from build123d import *

# Parameters (mm, degrees)
SKETCH1_W           = 4
SKETCH1_H           = 21
BOSS_EXTRUDE1_DEPTH = 4
CUT_EXTRUDE1_REACH  = 174.587
SKETCH3_W           = 34
SKETCH3_H           = 4
SKETCH3_W_2         = 46
SKETCH3_W_3         = 24


with BuildPart() as part:
    # Sketch1 → Boss-Extrude1 (new body)
    with BuildSketch(Plane(origin=(0, 0, 0), x_dir=(1, 0, 0), z_dir=(0, 1, 0))):
        with BuildLine():
            Line((-170, -29.5), (170, -29.5))
            Line((170, -29.5), (170, 29.5))
            Line((170, 29.5), (112, 29.5))
            Line((112, 29.5), (112, 25.5))
            Line((112, 25.5), (78, 25.5))
            Line((78, 25.5), (78, 29.5))
            Line((78, 29.5), (52.1, 29.5))
            Line((52.1, 29.5), (52.1, 27.5))
            ThreePointArc((52.1, 27.5), (50.5, 25.9), (48.9, 27.5))
            Line((48.9, 27.5), (48.9, 29.5))
            Line((48.9, 29.5), (23, 29.5))
            Line((23, 29.5), (23, 25.5))
            Line((23, 25.5), (-23, 25.5))
            Line((-23, 25.5), (-23, 29.5))
            Line((-23, 29.5), (-48.9, 29.5))
            Line((-48.9, 29.5), (-48.9, 27.5))
            ThreePointArc((-48.9, 27.5), (-50.5, 25.9), (-52.1, 27.5))
            Line((-52.1, 27.5), (-52.1, 29.5))
            Line((-52.1, 29.5), (-78, 29.5))
            Line((-78, 29.5), (-78, 25.5))
            Line((-78, 25.5), (-112, 25.5))
            Line((-112, 25.5), (-112, 29.5))
            Line((-112, 29.5), (-170, 29.5))
            Line((-170, 29.5), (-170, -29.5))
        make_face()
        with Locations((-148, -2)):
            Rectangle(SKETCH1_W, SKETCH1_H, mode=Mode.SUBTRACT)
        with Locations((148, -2)):
            Rectangle(SKETCH1_W, SKETCH1_H, mode=Mode.SUBTRACT)
    extrude(amount=BOSS_EXTRUDE1_DEPTH)

    # Sketch3 → Cut-Extrude1 (cut, up to next)
    with BuildSketch(Plane.XZ, mode=Mode.PRIVATE) as cut_extrude1_sk1:
        with Locations((-95, 27.5)):
            Rectangle(SKETCH3_W, SKETCH3_H)
    cut_extrude1_tool1 = extrude(cut_extrude1_sk1.sketch, amount=-CUT_EXTRUDE1_REACH, mode=Mode.PRIVATE) & part.part
    # Sketch3 → Cut-Extrude1 (cut, up to next)
    with BuildSketch(Plane.XZ, mode=Mode.PRIVATE) as cut_extrude1_sk2:
        with Locations((0, 27.5)):
            Rectangle(SKETCH3_W_2, SKETCH3_H)
    cut_extrude1_tool2 = extrude(cut_extrude1_sk2.sketch, amount=-CUT_EXTRUDE1_REACH, mode=Mode.PRIVATE) & part.part
    # Sketch3 → Cut-Extrude1 (cut, up to next)
    with BuildSketch(Plane.XZ, mode=Mode.PRIVATE) as cut_extrude1_sk3:
        with Locations((95, 27.5)):
            Rectangle(SKETCH3_W, SKETCH3_H)
    cut_extrude1_tool3 = extrude(cut_extrude1_sk3.sketch, amount=-CUT_EXTRUDE1_REACH, mode=Mode.PRIVATE) & part.part
    # Sketch3 → Cut-Extrude1 (cut, up to next)
    with BuildSketch(Plane.XZ, mode=Mode.PRIVATE) as cut_extrude1_sk4:
        with Locations((-158, -27.5)):
            Rectangle(SKETCH3_W_3, SKETCH3_H)
    cut_extrude1_tool4 = extrude(cut_extrude1_sk4.sketch, amount=-CUT_EXTRUDE1_REACH, mode=Mode.PRIVATE) & part.part
    # Sketch3 → Cut-Extrude1 (cut, up to next)
    with BuildSketch(Plane.XZ, mode=Mode.PRIVATE) as cut_extrude1_sk5:
        with Locations((158, -27.5)):
            Rectangle(SKETCH3_W_3, SKETCH3_H)
    cut_extrude1_tool5 = extrude(cut_extrude1_sk5.sketch, amount=-CUT_EXTRUDE1_REACH, mode=Mode.PRIVATE) & part.part
    add(cut_extrude1_tool1.solids().sort_by_distance((-95, 0, 27.5))[0], mode=Mode.SUBTRACT)
    add(cut_extrude1_tool2.solids().sort_by_distance((0, 0, 27.5))[0], mode=Mode.SUBTRACT)
    add(cut_extrude1_tool3.solids().sort_by_distance((95, 0, 27.5))[0], mode=Mode.SUBTRACT)
    add(cut_extrude1_tool4.solids().sort_by_distance((-158, 0, -27.5))[0], mode=Mode.SUBTRACT)
    add(cut_extrude1_tool5.solids().sort_by_distance((158, 0, -27.5))[0], mode=Mode.SUBTRACT)


solid = part.part
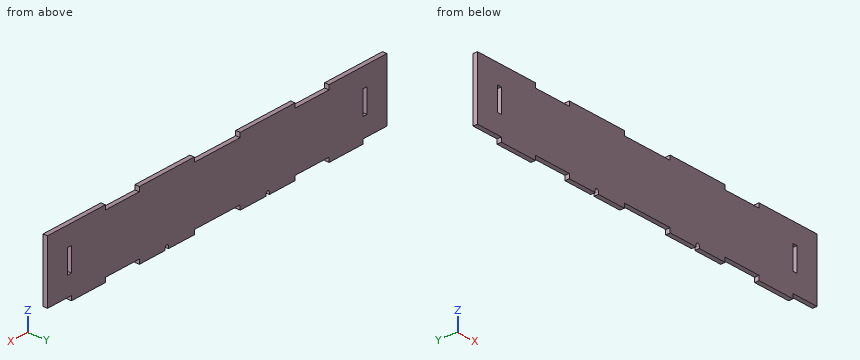
Read the model definition and answer for the solid it produces. Units are mm, in the model's axes. Coordinates: 2 decimals unless noted, no trailing zeros.
Q1. Consider probe 1 along X at (y, z) = (2.25, -6.5); probe 2 along Z at (x, y) = (-147, 3.4); probe 3 along Z at (x, y) = (-5.5, 0.55). Determine where each line is inside the solid, lowest interval first.
Q2. Each of these flat-tipped pins is pushed along its axis until it touches: pin 1 Ø1 at (y, z) = (1, -29) entering from -X; pin 2 Ø1 at (x, y) = (-16.5, 2.5) entering from -Z; pin 3 Ø10 at (x, z) = (81.5, -8.5) entering from -Y. Where does it stop, or does it pass through?
Q3. The part is cut by section A-A on y = 2.5. Give the number of separate pieces and of enclosed holes in the cut face, and give its area (3 significant figures).
Results below:
1. probe 1: x = -170 to -150, -146 to 146, 150 to 170
1. probe 2: z = -25.5 to -8.5, 12.5 to 29.5
1. probe 3: z = -25.5 to 25.5
2. pin 1: stops at x = -146
2. pin 2: stops at z = -25.5
2. pin 3: stops at y = 0
3. separate pieces: 1
3. enclosed holes: 2
3. area: 18,800 mm2
